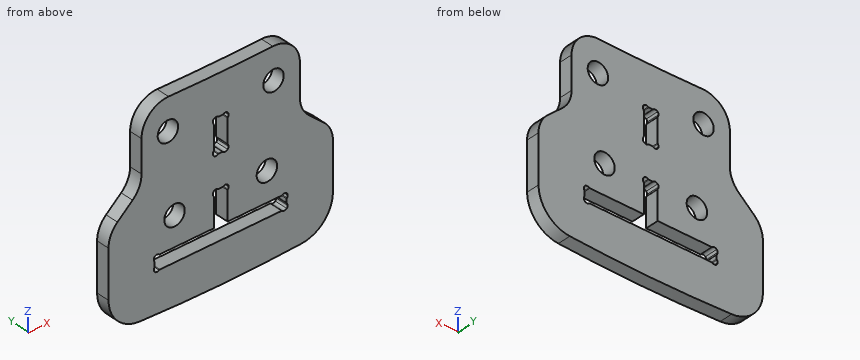
```python
from build123d import *

# Parameters (mm, degrees)
EXTRUDE_1_DEPTH     = 2
SKETCH_2_W          = 1.05
SKETCH_2_H          = 5.1
CUT_EXTRUDE_1_DEPTH = 343.228344823
CUT_EXTRUDE_2_DEPTH = 343.228344823
FILLET_1_R          = 0.2
SKETCH_4_R          = 1.55
CUT_EXTRUDE_3_DEPTH = 343.228344823
FILLET_2_R          = 5
FILLET_3_R          = 4


with BuildPart() as part:
    # 草图1 → 凸台-拉伸1 (new body)
    with BuildSketch(Plane(origin=(0, 0, 0), x_dir=(1, 0, 0), z_dir=(0, 1, 0))):
        with BuildLine():
            Line((-17, 327.5), (-12, 323.088235294))
            Line((-12, 323.088235294), (-12, 312.269515003))
            ThreePointArc((-12, 312.269515003), (0, 312.5), (12, 312.269515003))
            Line((12, 312.269515003), (12, 323.088235294))
            Line((12, 323.088235294), (17, 327.5))
            Line((17, 327.5), (17, 341.184299815))
            ThreePointArc((17, 341.184299815), (0, 341.8), (-17, 341.184299815))
            Line((-17, 341.184299815), (-17, 327.5))
        make_face()
    extrude(amount=EXTRUDE_1_DEPTH)

    # 草图2 → 切除-拉伸1 (cut, through all)
    with BuildSketch(Plane(origin=(0, 2, 0), x_dir=(1, 0, 0), z_dir=(0, 1, 0))):
        Polygon((0, 335.65), (0, 328.45), (1.05, 328.45), (1.05, 333.55), (10, 333.55), (10, 335.65), align=None)
        Polygon((-1.05, 328.45), (0, 328.45), (0, 335.65), (-10, 335.65), (-10, 333.55), (-1.05, 333.55), align=None)
        with Locations((0.525, 321.05)):
            Rectangle(SKETCH_2_W, SKETCH_2_H)
        with Locations((-0.525, 321.05)):
            Rectangle(SKETCH_2_W, SKETCH_2_H)
    extrude(amount=-CUT_EXTRUDE_1_DEPTH, mode=Mode.SUBTRACT)

    # 草图3 → 切除-拉伸2 (cut, through all)
    with BuildSketch(Plane(origin=(0, 2, 0), x_dir=(1, 0, 0), z_dir=(0, 1, 0))):
        with BuildLine():
            Line((10, 335.65), (10, 334.942893219))
            ThreePointArc((10, 334.942893219), (10.108386376, 335.105104893), (10.146446609, 335.296446609))
            ThreePointArc((10.146446609, 335.296446609), (10.108386376, 335.487788326), (10, 335.65))
        make_face()
        with BuildLine():
            ThreePointArc((10, 335.65), (9.646446609, 335.796446609), (9.292893219, 335.65))
            Line((9.292893219, 335.65), (10, 335.65))
        make_face()
        with BuildLine():
            ThreePointArc((10.146446609, 333.903553391), (10.108386376, 334.094895107), (10, 334.257106781))
            Line((10, 334.257106781), (10, 333.55))
            ThreePointArc((10, 333.55), (10.108386376, 333.712211674), (10.146446609, 333.903553391))
        make_face()
        with BuildLine():
            Line((10, 333.55), (9.292893219, 333.55))
            ThreePointArc((9.292893219, 333.55), (9.646446609, 333.403553391), (10, 333.55))
        make_face()
        with BuildLine():
            ThreePointArc((1.196446609, 328.803553391), (1.158386376, 328.994895107), (1.05, 329.157106781))
            Line((1.05, 329.157106781), (1.05, 328.45))
            ThreePointArc((1.05, 328.45), (1.158386376, 328.612211674), (1.196446609, 328.803553391))
        make_face()
        with BuildLine():
            Line((1.05, 328.45), (0.342893219, 328.45))
            ThreePointArc((0.342893219, 328.45), (0.696446609, 328.303553391), (1.05, 328.45))
        make_face()
        with BuildLine():
            ThreePointArc((1.196446609, 323.246446609), (1.158386376, 323.437788326), (1.05, 323.6))
            Line((1.05, 323.6), (1.05, 322.892893219))
            ThreePointArc((1.05, 322.892893219), (1.158386376, 323.055104893), (1.196446609, 323.246446609))
        make_face()
        with BuildLine():
            ThreePointArc((1.05, 323.6), (0.696446609, 323.746446609), (0.342893219, 323.6))
            Line((0.342893219, 323.6), (1.05, 323.6))
        make_face()
        with BuildLine():
            ThreePointArc((1.196446609, 318.853553391), (1.158386376, 319.044895107), (1.05, 319.207106781))
            Line((1.05, 319.207106781), (1.05, 318.5))
            ThreePointArc((1.05, 318.5), (1.158386376, 318.662211674), (1.196446609, 318.853553391))
        make_face()
        with BuildLine():
            Line((1.05, 318.5), (0.342893219, 318.5))
            ThreePointArc((0.342893219, 318.5), (0.696446609, 318.353553391), (1.05, 318.5))
        make_face()
    cut_extrude_2 = extrude(amount=-CUT_EXTRUDE_2_DEPTH, mode=Mode.SUBTRACT)

    # 镜向1: 切除-拉伸2 across plane
    add(cut_extrude_2.mirror(Plane(origin=(0, 0, 0), x_dir=(0, 0, 1), z_dir=(1, 0, 0))), mode=Mode.SUBTRACT)

    # 圆角1
    fillet_1_edges = [part.edges().sort_by_distance(p)[0] for p in [
        (1.05, 1, -329.157106781),
        (0.342893219, 1, -323.6),
        (1.05, 1, -319.207106781),
        (9.292893219, 1, -335.65),
        (10, 1, -334.257106781),
        (0.342893219, 1, -328.45),
        (1.05, 1, -322.892893219),
        (0.342893219, 1, -318.5),
        (-10, 1, -334.942893219),
        (-9.292893219, 1, -333.55),
        (-1.05, 1, -329.157106781),
        (-0.342893219, 1, -323.6),
        (-1.05, 1, -319.207106781),
        (-9.292893219, 1, -335.65),
        (-10, 1, -334.257106781),
        (-0.342893219, 1, -328.45),
        (-1.05, 1, -322.892893219),
        (-0.342893219, 1, -318.5),
        (10, 1, -334.942893219),
        (9.292893219, 1, -333.55),
    ]]
    fillet(fillet_1_edges, radius=FILLET_1_R)

    # 草图4 → 切除-拉伸3 (cut, through all)
    with BuildSketch(Plane(origin=(0, 2, 0), x_dir=(1, 0, 0), z_dir=(0, 1, 0))):
        with Locations(Location((7, 329.15, 0), (0, 0, 270))):
            Circle(SKETCH_4_R)
        with Locations(Location((8, 317.15, 0), (0, 0, 270))):
            Circle(SKETCH_4_R)
    cut_extrude_3 = extrude(amount=-CUT_EXTRUDE_3_DEPTH, mode=Mode.SUBTRACT)

    # 镜向2: 切除-拉伸3 across plane
    add(cut_extrude_3.mirror(Plane(origin=(0, 0, 0), x_dir=(0, 0, 1), z_dir=(1, 0, 0))), mode=Mode.SUBTRACT)

    # 圆角2
    fillet_2_edges = [part.edges().sort_by_distance(p)[0] for p in [
        (-17, 1, -341.184299815),
        (17, 1, -341.184299815),
    ]]
    fillet(fillet_2_edges, radius=FILLET_2_R)

    # 圆角3
    fillet_3_edges = [part.edges().sort_by_distance(p)[0] for p in [
        (17, 1, -327.5),
        (12, 1, -323.088235294),
        (12, 1, -312.269515003),
        (-12, 1, -312.269515003),
        (-12, 1, -323.088235294),
        (-17, 1, -327.5),
    ]]
    fillet(fillet_3_edges, radius=FILLET_3_R)


solid = part.part
```
The model under review builds one solid part; all positions refer to its coordinate system, in mm. Coordinates: 2 decimals unless noted, no trailing zeros. Write each loop counter-clockwise with the first axis right and the second up, starting at its lowest first coordinate (ties: lowest second). Pieces come first, ordered by that corner, then holes.
1) We need section A-A on z = -317.15. State the section outline as (x, y) points, then the cut area to 3 significant figures.
2) To check wall thickness, follow probe 1 along X at (y, z) = (0.9, -317.15); probe 2 along X at (y, z) = (0.65, -333); probe 3 along X at (y, z) = (1.45, -329.15). State the ranges of each line that lie inside material, in increasing order.
3) We need section B-B on x = -3. State the section outline as (y, z) points.
4) We need section C-C on x = 7. State the section outline as (y, z) points.
5) We need section D-D on y = 0.35. Count the separate pieces of the cut face and the enclosed holes in it, then the cut area to 3 significant figures.
6) Clearance check with flat-ended pins moving along their axes: pin 1 Ø0.6 at (y, z) = (0.5, -319.5) entering from +X; pin 2 Ø1 at (x, y) = (-4, 0.5) entering from +Z; pin 3 Ø2.5 at (x, z) = (-8, -317.15) entering from +Y. State where each tip first meets the part, or that it passes through.
Answer list:
1. outline: (-12, 0) - (-9.55, 0) - (-9.55, 2) - (-12, 2) - close; (-6.45, 0) - (6.45, 0) - (6.45, 2) - (-6.45, 2) - close; (9.55, 0) - (12, 0) - (12, 2) - (9.55, 2) - close
1. area: 35.6 mm2
2. probe 1: x = -12 to -9.55, -6.45 to 6.45, 9.55 to 12
2. probe 2: x = -17 to -1.05, 1.05 to 17
2. probe 3: x = -17 to -8.55, -5.45 to -1.07, 1.07 to 5.45, 8.55 to 17
3. outline: (0, -341.78) - (2, -341.78) - (2, -335.65) - (0, -335.65) - close; (0, -333.55) - (2, -333.55) - (2, -312.49) - (0, -312.49) - close
4. outline: (0, -341.7) - (2, -341.7) - (2, -335.65) - (0, -335.65) - close; (0, -333.55) - (2, -333.55) - (2, -330.7) - (0, -330.7) - close; (0, -327.6) - (2, -327.6) - (2, -318.33) - (0, -318.33) - close; (0, -315.97) - (2, -315.97) - (2, -312.42) - (0, -312.42) - close
5. separate pieces: 1
5. enclosed holes: 6
5. area: 751 mm2
6. pin 1: stops at x = 12
6. pin 2: stops at z = -312.47
6. pin 3: passes through
